```python
from build123d import *

# Parameters (mm, degrees)
SKETCH2_R          = 4
CUT_EXTRUDE1_DEPTH = 16
CIRPATTERN1_COUNT  = 6
CHAMFER1_SIZE      = 4
CHAMFER2_SIZE      = 4
FILLET1_R          = 4
FILLET2_R          = 4


with BuildPart() as part:
    # Sketch1 → Revolve1 (revolve)
    with BuildSketch(Plane.XY, mode=Mode.PRIVATE) as revolve1_sk:
        Polygon((24, -46.7154047), (36, -46.7154047), (36, -22.7154047), (27.164490862, -22.7154047), (27.164490862, -14.7154047), (54, -14.7154047), (54, 1.2845953), (27.164490862, 1.2845953), (27.164490862, 7.2845953), (36, 7.2845953), (36, 25.2845953), (24, 25.2845953), align=None)
    revolve(revolve1_sk.sketch.rotate(Axis((0, 63.408022787, 0), (0, -1, 0)), 90), axis=Axis((0, 63.408022787, 0), (0, -1, 0)))

    # Sketch2 → Cut-Extrude1 (cut)
    with BuildSketch(Plane(origin=(0, 1.2845953, 0), x_dir=(1, 0, 0), z_dir=(0, 1, 0))):
        with Locations(Location((0, 44, 0), (0, 0, 270))):
            Circle(SKETCH2_R)
    cut_extrude1 = extrude(amount=-CUT_EXTRUDE1_DEPTH, mode=Mode.SUBTRACT)

    # CirPattern1: Cut-Extrude1 ×6 about axis
    cirpattern1_axis = Axis((0, 0, 0), (0, 1, 0))
    for i in range(1, CIRPATTERN1_COUNT):
        add(cut_extrude1.rotate(cirpattern1_axis, i * 360 / CIRPATTERN1_COUNT), mode=Mode.SUBTRACT)

    # Chamfer1
    chamfer1_edges = [part.edges().sort_by_distance(p)[0] for p in [
        (0, 25.2845953, -36),
    ]]
    chamfer(chamfer1_edges, length=CHAMFER1_SIZE)

    # Chamfer2
    chamfer2_edges = [part.edges().sort_by_distance(p)[0] for p in [
        (0, -46.7154047, -36),
    ]]
    chamfer(chamfer2_edges, length=CHAMFER2_SIZE)

    # Fillet1
    fillet1_edges = [part.edges().sort_by_distance(p)[0] for p in [
        (0, -22.7154047, -27.164490862),
    ]]
    fillet(fillet1_edges, radius=FILLET1_R)

    # Fillet2
    fillet2_edges = [part.edges().sort_by_distance(p)[0] for p in [
        (0, 7.2845953, -27.164490862),
    ]]
    fillet(fillet2_edges, radius=FILLET2_R)


solid = part.part
```
For this review, take the finished solid that the model builds, in its own axes (mm). A direction names the side the tool comes from. Give positions to 0.01 mm unless a question says otherwise; leave off trailing zeros. Write each loop counter-clockwise with the first axis right and the second up, starting at its lowest first coordinate (ties: lowest second). Pieces come first, ordered by that corner, then holes. Notation, with made-up numbers: M -11.5,34.5 L 34.5,34.5 A19 cw 34.5,57.5 Z; hole C -2.5,-36 d9. An arc over 180 degrees is marked long. One line per item, written item: value.
1) For P1, Ø8, axis at x = -20.5, y = -15, coming from the +Z side; P2, Ø10.5, axis at x = 38.11, z = -22, coming from the +Y side; P3, Ø3, axis at y = -29, z = -31.5, coming from the -X side, all flat-tipped, find the tip position at first contact; note any pin that passes through.
Results are:
P1: stops at z = 51.41
P2: stops at y = 1.28
P3: stops at x = -19.9
2) Take a section at D-D, the plane z = -44. Write out the cut boundary in (x, y), then the cut area to 3 significant figures.
Results are:
outline: M -31.3,-14.72 L -4,-14.72 L -4,1.28 L -31.3,1.28 Z; M 4,-14.72 L 31.3,-14.72 L 31.3,1.28 L 4,1.28 Z
area: 874 mm²
3) For line 1 (Y direction, x = 7, z = 30); line 2 (Z direction, x = 1, y = 12.5); line 3 (X direction, y = -18, z = 0), list the stretches that pass through material, from the lowest coordinate up. Write a range as from..to.
Results are:
line 1: y = -46.72..-22.7, -14.72..1.28, 7.27..25.28
line 2: z = -35.99..-23.98, 23.98..35.99
line 3: x = -27.16..-24, 24..27.16
4) For faces 1 (the flat face through (-30, -22.715, -11)), 2 (the cylindrical face through (-24.331, -32.575, -26.533)), 3 (the cylindrical face through (-24.331, 14.383, -26.533)), list the 3-axis set-ups (+Z, -Z, +X, -X, +Y, -Y) from which the entire face can be reached by the end or side of a thin tool; tool diameter is ignored.
Results are:
face 1: none
face 2: -Y
face 3: +Y
5) Take a section at C-C, the plane y = -39. Write out the cut boundary in (x, z), then the cut area to 3 significant figures.
Results are:
outline: C 0,0 d72; hole C 0,0 d48
area: 2,260 mm²
6) The part is to be moulded in two halves that separate along X. For faces 4 (the cylindrical face through (2.4, -6.6, 47.2)), 5 (the flat face through (-13, 1.285, -25)), 6 (the cylindrical face through (52.716, -6.603, -11.706)), say which applies: +X half, -X half, draft (parallel to the pull), parting line (faces both ways), or undercut.
Results are:
face 4: undercut
face 5: draft
face 6: parting line
7) Take a section at B-B, the plane x = 39.5. Write out the cut boundary in (y, z), then the cut area to 3 significant figures.
Results are:
outline: M -14.72,-36.82 L 1.28,-36.82 L 1.28,-25.75 L -14.72,-25.75 Z; M -14.72,-18.25 L 1.28,-18.25 L 1.28,18.25 L -14.72,18.25 Z; M -14.72,25.75 L 1.28,25.75 L 1.28,36.82 L -14.72,36.82 Z
area: 938 mm²
